from build123d import *

# Parameters (mm, degrees)
F0_W     = 200
F0_H     = 200
F1_DEPTH = 300


with BuildPart() as f1:
    # F0 (on Top) → F1 (new body)
    with BuildSketch(Plane.XY):
        Rectangle(F0_W, F0_H)
    extrude(amount=F1_DEPTH)

    # F2 (on Right) → F3 (revolve, cut)
    with BuildSketch(Plane.YZ):
        with BuildLine():
            ThreePointArc((50, 300), (0, 350), (-50, 300))
            Line((-50, 300), (50, 300))
        make_face()
    revolve(axis=Axis((0, 0, 300), (0, 1, 0)), mode=Mode.SUBTRACT)


solid = f1.part
Here's how the part is built. I have some questions about the finished solid (model axes, mm). Coordinates: 2 decimals unless noted, no trailing zeros. Loops run counter-clockwise (first coordinate to the right, second up) from the corner with the lowest first, then second, coordinate; pieces in that order, holes last.
1. Imagine slicing it at B-B, the plane x = -42.5. Please give me the cut outline in (y, z).
2. I need wall thicknesses on L1, parallel to Z at x = 13, y = 13.5; L2, parallel to Z at x = -30.5, y = 12. Which ranges of each line are inside material? Lowest first, please.
3. Imagine slicing it at A-A, the plane y = -28. Please give me the cut outline in (x, z), and give its area (3 significant figures).
4. For P1, Ø4, axis at x = -27, y = -18.5, coming from the +Z side; P2, Ø2, axis at x = 32.5, y = -26.5, coming from the +Z side; P3, Ø1.5, axis at x = -14, y = -1, coming from the +Z side, each with a flat end and sliding along its axis, tell me the tip position at first contact or that it passes through.
Taken from the geometry:
1. outline: (-100, 0) - (100, 0) - (100, 300) - (26.34, 300) arc R26.34 cw to (-26.34, 300) - (-100, 300) - close
2. L1: z = 0 to 253.65
2. L2: z = 0 to 262.24
3. outline: (-100, 0) - (100, 0) - (100, 300) - (41.42, 300) arc R41.42 cw to (-41.42, 300) - (-100, 300) - close
3. area: 57,300 mm2
4. P1: stops at z = 264.03
4. P2: stops at z = 274.38
4. P3: stops at z = 252.24
